Model file for the job. Use its own axes, mm. Face numbers are marked on the shaded views. A direction names the side the tool comes from. Coordinates: 2 decimals unless noted, no trailing zeros. Order: outer loops, then holes, each group sorted by start corner. A loop starts at its lowest first (then second) coordinate and runs counter-clockwise, first axis right, second up. Notation, with made-up numbers: M 10,50.5 L 25,50.5 A17 cw 25,62.5 Z; hole C -10,16 d11. An arc over 180 degrees is marked long. Return JSON: item names as keys, results as strings.
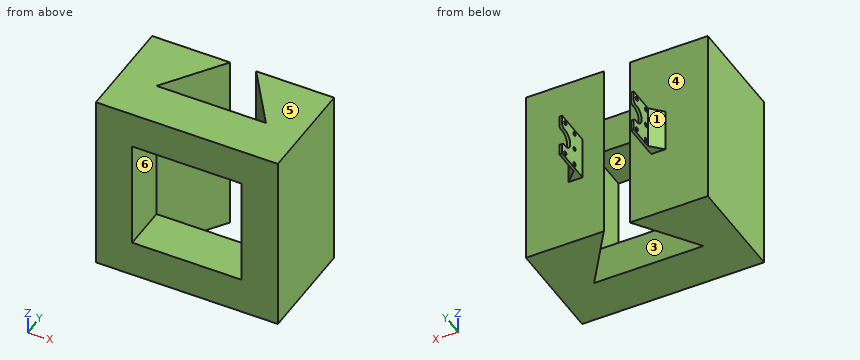
Autodesk Inventor part; units mm, degrees
ref_plane "XZ Plane" through (0, 0, 0) normal (0, 1, 0) x (-1, 0, 0)
ref_plane "XY Plane" through (0, 0, 0) normal (0, 0, 1) x (1, 0, 0)
sketch "Sketch1" plane through (0, 0, 0) normal (0, 1, 0) x (-1, 0, 0)
  line L0 (-38.25, 38.25) -> (38.25, 38.25)
  line L1 (38.25, 38.25) -> (38.25, -38.25)
  line L2 (38.25, -38.25) -> (-38.25, -38.25)
  line L3 (-38.25, -38.25) -> (-38.25, 38.25)
  line L4 (63.65, -63.65) -> (-63.65, -63.65)
  line L5 (-63.65, -63.65) -> (-63.65, 63.65)
  line L6 (-63.65, 63.65) -> (63.65, 63.65)
  line L7 (63.65, 63.65) -> (63.65, -63.65)
  point P0 (0, 0)
  point P1 (38.25, 0)
  point P2 (0, -38.25)
  point P3 (63.65, 0)
  point P4 (0, -63.65)
  dimension "d0" = 76.5
  dimension "d1" = 76.5
  dimension "d2" = 25.4
  dimension "d3" = 25.4
extrude "Extrusion1" add sketch "Sketch1" along normal blind 31.75
sketch "Sketch2" plane through (-63.65, 0, 63.65) normal (0, 0, 1) x (1, 0, 0)
  line L0 (127.3, 0) -> (127.3, 31.75) construction
  line L1 (0, 31.75) -> (127.3, 31.75) construction
  line L2 (101.9, 0) -> (101.9, 31.75) construction
  line L3 (101.9, 31.75) -> (72.7623, 73.3629)
  line L4 (101.9, 31.75) -> (152.7, 31.75) construction
  line L5 (63.65, 0) -> (63.65, 31.75)
  line L6 (72.7623, 73.3629) -> (127.3, 73.3629)
  line L7 (127.3, 73.3629) -> (127.3, 31.75)
  line L8 (25.4, 31.75) -> (54.5377, 73.3629)
  line L9 (25.4, 31.75) -> (-25.4, 31.75) construction
  line L10 (54.5377, 73.3629) -> (0, 73.3629)
  line L11 (0, 73.3629) -> (0, 31.75)
  line L12 (0, 31.75) -> (127.3, 31.75)
  dimension "d6" = 125
  dimension "d7" = 50.8
extrude "Extrusion2" add sketch "Sketch2" against normal up to surface (127.3 mm away)
sketch "Sketch3" plane through (9.1123, 73.3629, 63.65) normal (0, 1, 0) x (1, 0, 0)
  line L0 (-33.1123, 48.65) -> (-33.1123, 78.65)
  line L1 (-33.1123, 78.65) -> (-35.1123, 78.65)
  line L2 (-35.1123, 78.65) -> (-35.1123, 48.65)
  line L3 (-35.1123, 48.65) -> (-33.1123, 48.65)
  line L4 (16.8877, 48.65) -> (16.8877, 78.65)
  line L5 (16.8877, 78.65) -> (14.8877, 78.65)
  line L6 (14.8877, 78.65) -> (14.8877, 48.65)
  line L7 (14.8877, 48.65) -> (16.8877, 48.65)
  line L8 (-18.2246, 0) -> (-18.2246, 127.3) construction
  line L9 (-33.1123, 63.65) -> (14.8877, 63.65) construction
  point P0 (-9.1123, 63.65)
  point P1 (-18.2246, 63.65)
  point P2 (-9.1123, 63.65)
  dimension "d10" = 30
  dimension "d11" = 2
  dimension "d12" = 30
  dimension "d13" = 2
  dimension "d14" = 48
extrude "Extrusion3" add sketch "Sketch3" along normal blind 2
sketch "Sketch4" plane through (-26, 73.3629, 15) normal (-1, 0, 0) x (0, 0, 1)
  line L0 (0, 0) -> (-30, 0) construction
  line L1 (-30, 2) -> (0, 2) construction
  line L2 (0, 2) -> (-30, 2) construction
  line L3 (0, 2) -> (0, 26.5)
  line L4 (-30, 0) -> (0, 0) construction
  line L5 (0, 0) -> (-30, 0)
  line L6 (-30, 0) -> (-30, 2)
  line L7 (0, 0) -> (0, 2)
  line L8 (-30, 2) -> (0, 2)
  line L9 (-30, 2) -> (-30, 26.5)
  arc A0 (-21.25, 22.5) -> (-8.75, 22.5) centre (-15, 22.5) ccw
  line L10 (-21.25, 22.5) -> (-21.25, 24.5)
  line L11 (-8.75, 22.5) -> (-8.75, 24.5)
  line L12 (-30, 26.5) -> (-23.25, 26.5)
  line L13 (0, 26.5) -> (-6.75, 26.5)
  arc A1 (-21.25, 24.5) -> (-23.25, 26.5) centre (-23.25, 24.5) ccw
  arc A2 (-6.75, 26.5) -> (-8.75, 24.5) centre (-6.75, 24.5) ccw
  circle A3 centre (-3, 22.5) radius 1.4
  circle A4 centre (-3, 10.5) radius 1.4
  circle A5 centre (-15, 10.5) radius 1.4
  circle A6 centre (-27, 10.5) radius 1.4
  circle A7 centre (-27, 22.5) radius 1.4
  line L14 (-27, 10.5) -> (-15, 10.5) construction
  line L15 (-15, 10.5) -> (-3, 10.5) construction
  point P0 (-15, -73.3629)
  point P1 (-15, 2)
  point P2 (-15, 16.25)
  dimension "d17" = 26.5
  dimension "d18" = 12.5
  dimension "d19" = 22.5
  dimension "d20" = 2
  dimension "d21" = 2.8
  dimension "d22" = 12
  dimension "d23" = 24
extrude "Extrusion4" add sketch "Sketch4" against normal blind 2 contours L8 L9 L12 A1 L10 A0 L11 A2 L13 L3
sketch "Sketch5" plane through (-24, 73.3629, -15) normal (0, 0, -1) x (-1, 0, 0)
  line L0 (2, 0) -> (0, 0) construction
  line L1 (1, 8.89) -> (9.89, 0)
  line L2 (-14.8877, 0) -> (39.65, 0) construction
  line L3 (1, 8.89) -> (13.5724, 8.89) construction
  line L4 (1, 8.89) -> (-7.89, 0)
  line L5 (1, 8.89) -> (13.5724, 8.89) construction
  line L6 (1, 8.89) -> (1, 0)
  line L7 (1, 0) -> (9.89, 0)
  point P0 (-24, -73.3629)
  dimension "d26" = 45
  dimension "d27" = 135
  dimension "d28" = 8.89
extrude "Extrusion5" add sketch "Sketch5" against normal up to surface (30 mm away)
mirror "Mirror1" about plane through (0, 0, 0) normal (1, 0, 0) of "Extrusion4", "Extrusion5"
properties part number "ADAPTER4BB"
Item 1: Saw through at D-D (x = 50). Write the cut outline in (y, z), and give its area (3 significant figures).
Check result:
{"outline": "M 0,-63.65 L 73.36,-63.65 L 73.36,63.65 L 0,63.65 Z", "area": "9,340 mm2"}
Item 2: Saw through at B-B (x = -28). Write the cut outline in (y, z), and give its area (3 significant figures).
Check result:
{"outline": "M 0,-63.65 L 31.75,-63.65 L 31.75,-38.25 L 0,-38.25 Z; M 0,38.25 L 31.75,38.25 L 31.75,63.65 L 0,63.65 Z; M 46.39,-63.65 L 73.36,-63.65 L 73.36,-15 L 79.25,-15 L 79.25,15 L 73.36,15 L 73.36,63.65 L 46.39,63.65 Z", "area": "5,220 mm2"}
Item 3: Pull direction Z, two halves, no side cores. Call the marked faces 4, 5 and 6: +Z half, -Z half, draft (parallel to the pull), parting line (faces both ways), or undercut.
Check result:
{"face 4": "draft", "face 5": "+Z half", "face 6": "undercut"}
Item 4: 3-axis set-ups, long thin cutter, end or side, ignore diameter. For the marked faces 1, 2 and 3: which of +Z, -Z, +X, -X, +Y, -Y reach the whole face in a straight line?
Check result:
{"face 1": "+Z, -Z, -X, +Y", "face 2": "-Y", "face 3": "+Z, -Z"}
Item 5: Wall check: line 1 (Z direction, x = -7.5, y = 21.5); line 2 (Y direction, x = -56, z = -9.5). Give the ranges that are in metal, low to high.
Check result:
{"line 1": "z = -63.65 to -38.25, 38.25 to 63.65", "line 2": "y = 0 to 73.36"}
Item 6: Drop flat-ended pins along their axis: pin 1 Ø1 at (x, y) = (24.5, 97) entering from +Z; pin 2 Ø1.7 at (y, z) = (83.86, -12) entering from -X; pin 3 Ø0.6 at (x, y) = (25.5, 96.5) entering from -Z; pin 4 Ø1 at (x, z) = (37.5, -19.5) entering from +Y. Give the stop position or say it passes through.
Check result:
{"pin 1": "stops at z = 15", "pin 2": "passes through", "pin 3": "stops at z = -15", "pin 4": "stops at y = 73.36"}
Item 7: Saw through at A-A (z = -18.5). Write the cut outline in (x, y), and give its area (3 significant figures).
Check result:
{"outline": "M -63.65,0 L -38.25,0 L -38.25,31.75 L -9.11,73.36 L -63.65,73.36 Z; M 9.11,73.36 L 38.25,31.75 L 38.25,0 L 63.65,0 L 63.65,73.36 Z", "area": "4,940 mm2"}
Item 8: Saw through at C-C (y = 59). Write the cut outline in (x, z).
Check result:
{"outline": "M -63.65,-63.65 L -19.17,-63.65 L -19.17,63.65 L -63.65,63.65 Z; M 19.17,-63.65 L 63.65,-63.65 L 63.65,63.65 L 19.17,63.65 Z"}
